The listing builds one solid part. Answer for the finished solid, in the listing's coordinates (mm). A direction names the side the tool comes from. Coordinates: 2 decimals unless noted, no trailing zeros. Loops run counter-clockwise (first coordinate to the right, second up) from the corner with the lowest first, then second, coordinate; pieces in that order, holes last. Notation, with made-up numbers: M -2,-23 L 50,-23 A13 ccw 50,-1 Z; hole C -12.75,1.25 d4. An arc over 180 degrees is marked long. Answer as a JSON object with one key per item and string values. Group by question number.
1. Determine the mould class of faces 1 (the face through (69, -30, 18)), 2 (the face through (9, -43, -34)), 3 (the face through (6, -26, 23)), 4 (the face through (8.957, -44.479, 24.362)) for opening direction Z: released by +Z, released by -Z, zero draft, split by the parting line, or undercut.
2. A cutting plane is placed at B-B on z = 0. Give the vertices of the cut face in (x, y).
3. For faces 5 (the face through (66, -5, 0)), 6 (the face through (37, -10, 4)), 7 (the face through (68.9, -46, 31.4)), determine the directions among +Z, -Z, +X, -X, +Y, -Y from which every point of the face is accessible in a straight line to the end or side of a thin tool.
4. A cutting plane is placed at C-C on x = 15. Give the vertices of the cut face in (y, z).
5. Given pin 1 (18.5 mm diameter, centred on y = -23, z = -30.5, fed in from +X); pin 2 (3.5 mm diameter, centred on x = 71, z = 29, fed in from +Y); pin 3 (8 mm diameter, centred on x = 58.5, y = -2.5, fed in from +Z); pin 4 (9.5 mm diameter, centred on x = 9, y = -27, fed in from -Z), each flat-ended and moving along its own axis, determine where each tip first touches the part or whether it passes through.
6. Straight lines are drawn through the part: L1, parallel to X at y = -47, z = -29; L2, parallel to Z at x = 69, y = -47; L3, parallel to Z at x = 69, y = -45. For each, find the intervals that lie inside material, in ascending order.
7. A cutting plane is placed at D-D on x = 69. State how many separate pieces and enclosed holes the cut face has, and give its area (3 significant figures).
8. A cutting plane is placed at A-A on y = -45. Give the vertices of the cut face in (x, z).
from build123d import *

# Parameters (mm, degrees)
STRUCTURE_W                                     = 75
STRUCTURE_H                                     = 18
BOSS_CORPS_DEPTH                                = 10
BOSS_PATES_OUTLINE_W                            = 50
BOSS_PATES_OUTLINE_H                            = 5
BOSS_PATES_DEPTH                                = 12
BOSS_PATES_START                                = 63
BOSS_PATES_2_OUTLINE_W                          = 50
BOSS_PATES_2_OUTLINE_H                          = 5
BOSS_PATES_2_DEPTH                              = 12
SKETCH2_W                                       = 12
SKETCH2_H                                       = 7
BOSS_ATTACHES_DEPTH                             = 12
F_6_CLEARANCE_HOLE1_D                           = 4.3053
CBORE_FOR_6_PAN_HEAD_MACHINE_SCREW1_D           = 4.3053
CBORE_FOR_6_PAN_HEAD_MACHINE_SCREW1_CBORE_D     = 11.0000034
CBORE_FOR_6_PAN_HEAD_MACHINE_SCREW1_CBORE_DEPTH = 2.999994
FILLET1_R                                       = 8
CUT_EXTRUDE1_REACH                              = 98.695
SKETCH10_W                                      = 15
SKETCH10_H                                      = 20


# Read off the part's stored shape, not the designer's step: Boss-Pates
with BuildPart() as part:
    # Structure → Boss-Corps (new body)
    with BuildSketch(Plane(origin=(0, 0, 0), x_dir=(1, 0, 0), z_dir=(0, 1, 0))):
        with Locations((37.5, 9)):
            Rectangle(STRUCTURE_W, STRUCTURE_H)
    extrude(amount=-BOSS_CORPS_DEPTH)

    # Boss-Pates outline → Boss-Pates (add)
    with BuildSketch(Plane.YZ):
        with Locations((-25, -20.5)):
            Rectangle(BOSS_PATES_OUTLINE_W, BOSS_PATES_OUTLINE_H)
    extrude(amount=BOSS_PATES_DEPTH)

    # Boss-Pates 2 outline → Boss-Pates 2 (add)
    with BuildSketch(Plane.YZ.offset(BOSS_PATES_START)):
        with Locations((-25, -20.5)):
            Rectangle(BOSS_PATES_2_OUTLINE_W, BOSS_PATES_2_OUTLINE_H)
    extrude(amount=BOSS_PATES_2_DEPTH)

    # Sketch2 → Boss-Attaches (add)
    with BuildSketch(Plane(origin=(0, 0, -23), x_dir=(-1, 0, 0), z_dir=(0, 0, -1))):
        with Locations((-69, -46.5)):
            Rectangle(SKETCH2_W, SKETCH2_H)
        with Locations((-6, -46.5)):
            Rectangle(SKETCH2_W, SKETCH2_H)
    extrude(amount=BOSS_ATTACHES_DEPTH)

    # Mirror4: part across plane


with BuildPart() as part_1:
    add(part.part)
    add(part.part.mirror(Plane(origin=(0, -10, 0), x_dir=(1, 0, 0), z_dir=(0, 0, 1))))

    # #6 Clearance Hole1 (through all)
    with Locations(Plane(origin=(0, 0, 0), x_dir=(1, 0, 0), z_dir=(0, 1, 0))):
        with Locations((15, 0), (39, 0)):
            Hole(F_6_CLEARANCE_HOLE1_D / 2)

    # CBORE for #6 Pan Head Machine Screw1 (through all)
    with Locations(Plane(origin=(0, -43, 0), x_dir=(1, 0, 0), z_dir=(0, 1, 0))):
        with Locations((6, 29), (69, 29), (69, -29), (6, -29)):
            CounterBoreHole(CBORE_FOR_6_PAN_HEAD_MACHINE_SCREW1_D / 2, CBORE_FOR_6_PAN_HEAD_MACHINE_SCREW1_CBORE_D / 2, CBORE_FOR_6_PAN_HEAD_MACHINE_SCREW1_CBORE_DEPTH)

    # Fillet1
    fillet1_edges = [part_1.edges().sort_by_distance(p)[0] for p in [
        (69, 0, -23),
        (6, 0, 23),
    ]]
    fillet(fillet1_edges, radius=FILLET1_R)

    # Sketch10 → Cut-Extrude1 (cut, up to next)
    with BuildSketch(Plane(origin=(0, 0, 0), x_dir=(1, 0, 0), z_dir=(0, 1, 0)), mode=Mode.PRIVATE) as cut_extrude1_sk1:
        with Locations((58.5, 0)):
            Rectangle(SKETCH10_W, SKETCH10_H)
    cut_extrude1_tool1 = extrude(cut_extrude1_sk1.sketch, amount=-CUT_EXTRUDE1_REACH, mode=Mode.PRIVATE) & part_1.part
    add(cut_extrude1_tool1.solids().sort_by_distance((58.5, 0, 0))[0], mode=Mode.SUBTRACT)


solid = part_1.part
From the geometry:
{
 "1": {"face 1": "undercut", "face 2": "zero draft", "face 3": "released by +Z", "face 4": "undercut"},
 "2": {"outline": "M 0,-10 L 12.85,-10 L 12.85,0 L 0,0 Z; M 17.15,-10 L 36.85,-10 L 36.85,0 L 17.15,0 Z; M 41.15,-10 L 51,-10 L 51,0 L 41.15,0 Z; M 66,-10 L 75,-10 L 75,0 L 66,0 Z"},
 "3": {"face 5": "+Y, -Y", "face 6": "+X, -X, -Y", "face 7": "+Y"},
 "4": {"outline": "M -10,-18 L -0.58,-18 A8 ccw 0,-15 L 0,-2.15 L -10,-2.15 Z; M -10,2.15 L 0,2.15 L 0,15 A8 ccw -0.58,18 L -10,18 Z"},
 "5": {"pin 1": "stops at x = 75", "pin 2": "stops at y = -46", "pin 3": "stops at z = 18", "pin 4": "stops at z = -23"},
 "6": {"L1": "x = 0 to 3.85, 8.15 to 12, 63 to 66.85, 71.15 to 75", "L2": "z = -35 to -31.15, -26.85 to -18, 18 to 26.85, 31.15 to 35", "L3": "z = -35 to -34.5, -23.5 to -18, 18 to 23.5, 34.5 to 35"},
 "7": {"separate pieces": "3", "enclosed holes": "0", "area": "900 mm²"},
 "8": {"outline": "M 0,-35 L 12,-35 L 12,-18 L 0,-18 Z; M 0,18 L 12,18 L 12,35 L 0,35 Z; M 63,-35 L 75,-35 L 75,-18 L 63,-18 Z; M 63,18 L 75,18 L 75,35 L 63,35 Z; hole C 6,-29 d11; hole C 6,29 d11; hole C 69,-29 d11; hole C 69,29 d11"}
}
